Geometry check sheet. Reference: the model listing, model coordinates, mm. Face numbers are marked on the shaded views. A direction names the side the tool comes from. Coordinates: 2 decimals unless noted, no trailing zeros. Loops run counter-clockwise (first coordinate to the right, second up) from the corner with the lowest first, then second, coordinate; pieces in that order, holes last.
from build123d import *

# Parameters (mm, degrees)
SKETCH086_W     = 21
SKETCH086_H     = 4
PAD052_DEPTH    = 3
PAD053_DEPTH    = 32
SKETCH088_R     = 2.75
POCKET027_DEPTH = 5.001
SKETCH089_R     = 1.5
POCKET028_DEPTH = 5.001


with BuildPart() as part:
    # Sketch086 → Pad052 (new body)
    with BuildSketch(Plane.XY):
        with BuildLine():
            Line((-17.5, 18), (13.5, 18))
            ThreePointArc((17.5, 14), (16.328427, 16.828427), (13.5, 18))
            Line((17.5, 14), (17.5, -18))
            Line((17.5, -18), (-17.5, -18))
            Line((-17.5, -18), (-17.5, 18))
        make_face()
        with Locations((3, -10)):
            Rectangle(SKETCH086_W, SKETCH086_H, mode=Mode.SUBTRACT)
    extrude(amount=PAD052_DEPTH)

    # Sketch087 → Pad053 (join)
    with BuildSketch(Plane(origin=(0, 0, 0), x_dir=(-1, 0, 0), z_dir=(0, 0, -1))):
        Polygon((17.5, 18), (-2.5, 18), (-2.5, 13), (12.5, 13), (12.5, -1.7), (8.5, -1.7), (8.5, -2.7), (12.5, -2.7), (12.5, -17), (8.5, -17), (8.5, -18), (17.5, -18), align=None)
    extrude(amount=PAD053_DEPTH)

    # Sketch088 (on Face16 of Pad053) → Pocket027 (cut, through all)
    with BuildSketch(Plane.XZ.offset(-13)):
        with Locations((-7.5, -16)):
            Circle(SKETCH088_R)
    extrude(amount=-POCKET027_DEPTH, mode=Mode.SUBTRACT)

    # Sketch089 (on Face11 of Pocket027) → Pocket028 (cut, through all)
    with BuildSketch(Plane.YZ.offset(-12.5)):
        with Locations((-9.85, -24.55)):
            Circle(SKETCH089_R)
    extrude(amount=-POCKET028_DEPTH, mode=Mode.SUBTRACT)


solid = part.part
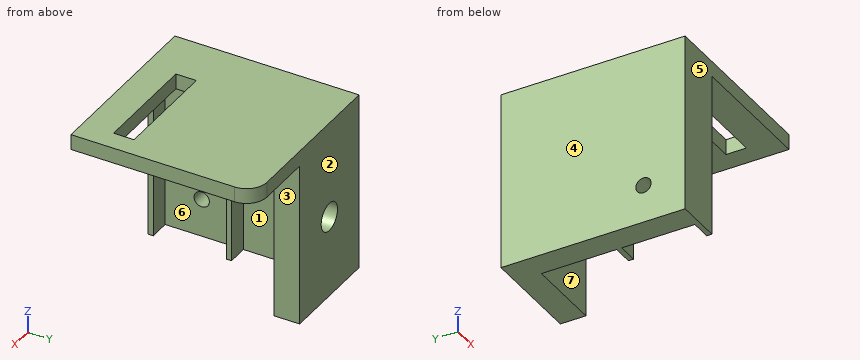
(1) Sectioned sample at C-C on x = 8. Record the cut outline in (y, z).
Findings:
outline: (-18, 0) - (-12, 0) - (-12, 3) - (-18, 3) - close; (-8, 0) - (18, 0) - (18, 3) - (-8, 3) - close
(2) Gauge pin test, flat ends, axial feed: pin 1 Ø4.5 at (y, z) = (-9.5, -20.5) entering from +X; pin 2 Ø2 at (x, y) = (6.5, 5) entering from -Z; pin 3 Ø5.5 at (y, z) = (15, -13) entering from +X. Record the tip position at first contact, or that the pin passes through.
Findings:
pin 1: stops at x = -12.5
pin 2: stops at z = 0
pin 3: stops at x = 2.5
(3) Access from +Z, -Z, +X, -X, +Y, -Y to the whole of each face (thin tool, end or side, straight path). Record for the marked faces 1, 2 and 3.
Findings:
face 1: -Z, +X
face 2: +Z, -Z, +X, -X, +Y
face 3: -Z, +X, +Y, -Y
(4) Sectioned sample at A-A on y = -9.85. Record the cut outline in (x, z), and give its area (3 significant figures).
Findings:
outline: (-17.5, -32) - (-12.5, -32) - (-12.5, -26.05) - (-17.5, -26.05) - close; (-17.5, -23.05) - (-12.5, -23.05) - (-12.5, 0) - (-7.5, 0) - (-7.5, 3) - (-17.5, 3) - close; (13.5, 0) - (17.5, 0) - (17.5, 3) - (13.5, 3) - close
area: 187 mm2
(5) Sectioned sample at D-D on x = -12. Record the cut outline in (y, z).
Findings:
outline: (-18, -32) - (-17, -32) - (-17, 0) - (-2.7, 0) - (-2.7, -32) - (-1.7, -32) - (-1.7, 0) - (13, 0) - (13, -32) - (18, -32) - (18, 3) - (-18, 3) - close
(6) Sectioned sample at B-B on z = -16. Record the cut outline in (x, y).
Findings:
outline: (-17.5, -18) - (-8.5, -18) - (-8.5, -17) - (-12.5, -17) - (-12.5, -2.7) - (-8.5, -2.7) - (-8.5, -1.7) - (-12.5, -1.7) - (-12.5, 13) - (-10.25, 13) - (-10.25, 18) - (-17.5, 18) - close; (-4.75, 13) - (2.5, 13) - (2.5, 18) - (-4.75, 18) - close
(7) Scan lines: L1, parallel to Y at x = -10, z = -24; L2, parallel to X at y = -1, z = -12; L3, parallel to Z at x = -7.5, y = 16.1. Record each from-to range of solid material in increasing order.
Findings:
L1: y = -18 to -17, -2.7 to -1.7, 13 to 18
L2: x = -17.5 to -12.5
L3: z = -32 to -18.75, -13.25 to 3
(8) Draft check along Y on the marked faces 4, 5, 6 and 7. Enter one of: +Y half, -Y half, draft (parallel to the pull), parting line (faces both ways), or undercut.
Findings:
face 4: draft
face 5: -Y half
face 6: undercut
face 7: undercut
